Here's how the part is built. I have some questions about the finished solid (model axes, mm). Face numbers are marked on the shaded views. A direction names the side the tool comes from. Coordinates: 2 decimals unless noted, no trailing zeros. Order: outer loops, then holes, each group sorted by start corner. A loop starts at its lowest first (then second) coordinate and runs counter-clockwise, first axis right, second up. Notation, with made-up numbers: (69, 66) - (93, 66) arc R28 ccw to (93, 102) - close; hole circle Ø7 at (32, 77.25). An arc over 180 degrees is marked (long way). Use CSV: the item, a comma, the result in double quotes. Start each with the question number.
from build123d import *

# Parameters (mm, degrees)
F0_R     = 5.5
F1_DEPTH = 9
F2_W     = 59
F2_H     = 9
F3_DEPTH = 9
F5_DEPTH = 9


with BuildPart() as f1:
    # F0 (on Top) → F1 (new body)
    with BuildSketch(Plane.XY):
        with BuildLine():
            Line((59, 0), (0, 0))
            Line((0, 0), (0, -15))
            ThreePointArc((0, -15), (3.8076118446, -24.1923881554), (13, -28))
            Line((13, -28), (46, -28))
            ThreePointArc((46, -28), (55.1923881554, -24.1923881554), (59, -15))
            Line((59, -15), (59, 0))
        make_face()
        with Locations((13, -15)):
            Circle(F0_R, mode=Mode.SUBTRACT)
        with Locations((46, -15)):
            Circle(F0_R, mode=Mode.SUBTRACT)
    extrude(amount=-F1_DEPTH)

    # F2 (on face) → F3 (join)
    with BuildSketch(Plane(origin=(0, 0, 0), x_dir=(-1, 0, 0), z_dir=(0, 1, 0))):
        with Locations((-29.5, -4.5)):
            Rectangle(F2_W, F2_H)
        Polygon((0, 0), (-68, 68), (-90.627416998, 45.372583002), (-59, 0), align=None)
    extrude(amount=F3_DEPTH)

    # F4 (on face) → F5 (join)
    with BuildSketch(Plane(origin=(68, 0, 68), x_dir=(0, 1, 0), z_dir=(0.7071067812, 0, 0.7071067812))):
        with BuildLine():
            Line((0, -32), (0, 0))
            Line((0, 0), (-20, 0))
            Line((-20, 0), (-20, -9))
            ThreePointArc((-20, -9), (-15.0502525317, -11.0502525317), (-13, -16))
            ThreePointArc((-13, -16), (-15.0502525317, -20.9497474683), (-20, -23))
            Line((-20, -23), (-20, -32))
            Line((-20, -32), (0, -32))
        make_face()
        with BuildLine():
            Line((-20, -9), (-20, 0))
            ThreePointArc((-20, 0), (-36, -16), (-20, -32))
            Line((-20, -32), (-20, -23))
            ThreePointArc((-20, -23), (-27, -16), (-20, -9))
        make_face()
    extrude(amount=-F5_DEPTH)


solid = f1.part
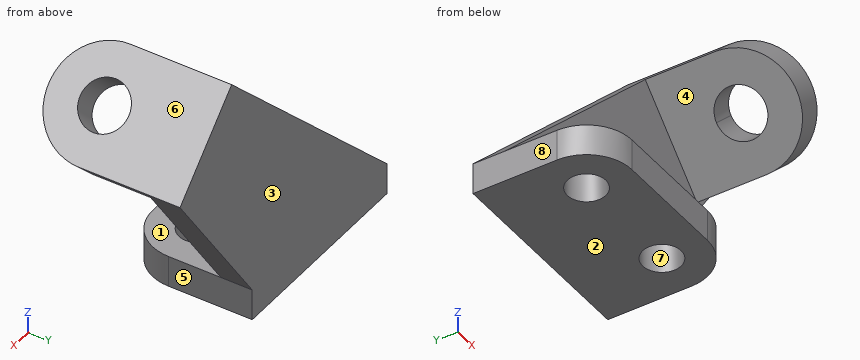
Item 1: Suppose I cut it at B-B on x = 49. Write out the boundary of the cut face in (y, z).
Item 2: Suppose I cut it at A-A on y = -1.5. Write out the boundary of the cut face in (x, z), then the cut area to 3 significant figures.
Item 3: We'd pull the mould along X, two halves only. Please class the marked faces 6, 7 and 8: released by +X, released by -X, zero draft, split by the parting line, or undercut.
Item 4: For pin 1 Ø6 at (y, z) = (-18, 58.5) entering from -X; pin 2 Ø5 at (x, z) = (51.5, 18) entering from -Y; pin 3 Ø9 at (x, y) = (46, -15) entering from +Z; pin 4 Ø5 at (y, z) = (-0.5, 38.5) entering from +X, each with a flat end and sliding along its axis, tell me the tip position at first contact or that it passes through.
Item 5: Suppose I cut it at C-C on y = -17.5. Write out the boundary of the cut face in (x, z).
Item 6: For the marked faces 1, 2, 3, 4 and 5, which set-ups out of +Z, -Z, +X, -X, +Y, -Y let a thin tool reach every point of the face, with its end or its side?
Item 7: Please list where these lines run through material, in increasing order: line 1 along Y through (x, z) = (46, -6.5); line 2 along Z through (x, y) = (49, -27.5); line 3 along Y through (x, z) = (23.5, -0.5). Write a range as from..to.
Item 8: Suppose I cut it at D-D on x = 31.5. Write out the boundary of the cut face in (y, z), then the cut area to 4 significant figures.
Here are the results:
1,outline,"(-27.65, -9) - (-19.61, -9) - (-19.61, 0) - (-27.65, 0) - close; (-10.39, -9) - (9, -9) - (9, 49) - (0, 49) - (0, 0) - (-10.39, 0) - close"
2,outline,"(0, -9) - (59, -9) - (59, 0) - (0, 0) - close; (61.64, 61.64) - (84.26, 39.01) - (90.63, 45.37) - (68, 68) - close"
2,area,"819 mm^2"
3,face 6,"released by +X"
3,face 7,"undercut"
3,face 8,"released by -X"
4,pin 1,"x = 61.77"
4,pin 2,"y = 0"
4,pin 3,"through"
4,pin 4,"x = 87.54"
5,outline,"(0.24, -9) - (8.1, -9) - (8.1, 0) - (0.24, 0) - close; (17.9, -9) - (41.1, -9) - (41.1, 0) - (17.9, 0) - close; (50.9, -9) - (58.76, -9) - (58.76, 0) - (50.9, 0) - close; (61.64, 61.64) - (68.33, 54.95) - (74.69, 61.31) - (68, 68) - close; (77.57, 45.7) - (84.26, 39.01) - (90.63, 45.37) - (83.94, 52.06) - close"
6,face 1,"+Z, +X, -X, -Y"
6,face 2,"-Z, +X, -X, +Y, -Y"
6,face 3,"+Z, -Z, +X, -X, +Y"
6,face 4,"-Z, -X, -Y"
6,face 5,"-Z, +X, +Y, -Y"
7,line 1,"-28..-20.5, -9.5..9"
7,line 2,"-9..0"
7,line 3,"-28..9"
8,outline,"(-28, -9) - (9, -9) - (9, 31.5) - (0, 31.5) - (0, 0) - (-28, 0) - close"
8,area,"616.5 mm^2"
